For this review, take the finished solid that the model builds, in its own axes (mm). Round coordinates to 2 decimals unless told otherwise and drop trailing zeros. Write each loop counter-clockwise with the first axis right and the second up, starting at its lowest first coordinate (ties: lowest second). Pieces come first, ordered by that corner, then holes. Notation, with made-up numbers: (66.5, 41) - (121.5, 41) arc R28 ccw to (121.5, 60) - close; hole circle Ø3 at (-7, 89). An arc over 180 degrees is marked (long way). One line per item, written item: value. Start each with the question number.
Q1. Add section B-B on z = 3.6. Write out the cut boundary in (x, y).
Q2. Add section C-C on y = 11. Write out the cut boundary in (x, z), and give its area (3 significant figures).
Q3. Add section A-A on x = -15.56. Write out the cut boundary in (y, z), and give its area (3 significant figures).
Q4. Add section D-D on x = -30.56. Write out the cut boundary in (y, z), and give its area (3 significant figures).
Q5. For probe 1 along Y at (x, z) = (32.06, 2.95); probe 2 along X at (y, z) = (6, 2.35); probe 3 along Y at (x, z) = (-30.56, 3.15), list the stretches that pass through material, from the lowest coordinate up.
Q6. Mouldability with a two-part tool opening along Y and no side actions: class faces 1 (the face through (-34.65, 11.99, 2.41)), 2 (the face through (-34.65, -11.99, 2.41)), 3 (the face through (-32.06, 5.15, 2.41)) as +Y half, -Y half, draft (parallel to the pull), parting line (faces both ways), or undercut.
```python
from build123d import *

# Parameters (mm, degrees)
ESQUISSE1_W             = 75
ESQUISSE1_H             = 30
BOSS_EXTRU_1_DEPTH      = 4.7625
CONG_1_R                = 10
ESQUISSE3_R             = 1.5
ENL_V_MAT_EXTRU_3_DEPTH = 10


with BuildPart() as part:
    # Esquisse1 → Boss.-Extru.1 (new body)
    with BuildSketch(Plane.XY):
        Rectangle(ESQUISSE1_W, ESQUISSE1_H)
    extrude(amount=BOSS_EXTRU_1_DEPTH)

    # Congé1
    cong_1_edges = [part.edges().sort_by_distance(p)[0] for p in [
        (-37.5, -15, 2.38125),
        (-37.5, 15, 2.38125),
    ]]
    fillet(cong_1_edges, radius=CONG_1_R)

    # Esquisse3 → Enlèv. mat.-Extru.3 (cut)
    with BuildSketch(Plane.XY.offset(4.7625)):
        with Locations((-15.56, 5.08)):
            Circle(ESQUISSE3_R)
        with Locations((-15.56, -5.08)):
            Circle(ESQUISSE3_R)
        with Locations((32.06, -5.08)):
            Circle(ESQUISSE3_R)
        with Locations((32.06, 5.08)):
            Circle(ESQUISSE3_R)
        with Locations((-30.56, 5.08)):
            Circle(ESQUISSE3_R)
        with Locations((-30.56, -5.08)):
            Circle(ESQUISSE3_R)
    extrude(amount=-ENL_V_MAT_EXTRU_3_DEPTH, mode=Mode.SUBTRACT)


solid = part.part
```
Result set:
1. outline: (-37.5, -5) arc R10 ccw to (-27.5, -15) - (37.5, -15) - (37.5, 15) - (-27.5, 15) arc R10 ccw to (-37.5, 5) - close; hole circle Ø3 at (-30.56, -5.08); hole circle Ø3 at (-30.56, 5.08); hole circle Ø3 at (-15.56, -5.08); hole circle Ø3 at (-15.56, 5.08); hole circle Ø3 at (32.06, -5.08); hole circle Ø3 at (32.06, 5.08)
2. outline: (-35.5, 0) - (37.5, 0) - (37.5, 4.76) - (-35.5, 4.76) - close
2. area: 348 mm^2
3. outline: (-15, 0) - (-6.58, 0) - (-6.58, 4.76) - (-15, 4.76) - close; (-3.58, 0) - (3.58, 0) - (3.58, 4.76) - (-3.58, 4.76) - close; (6.58, 0) - (15, 0) - (15, 4.76) - (6.58, 4.76) - close
3. area: 114 mm^2
4. outline: (-14.52, 0) - (-6.58, 0) - (-6.58, 4.76) - (-14.52, 4.76) - close; (-3.58, 0) - (3.58, 0) - (3.58, 4.76) - (-3.58, 4.76) - close; (6.58, 0) - (14.52, 0) - (14.52, 4.76) - (6.58, 4.76) - close
4. area: 110 mm^2
5. probe 1: y = -15 to -6.58, -3.58 to 3.58, 6.58 to 15
5. probe 2: x = -37.45 to -31.74, -29.38 to -16.74, -14.38 to 30.88, 33.24 to 37.5
5. probe 3: y = -14.52 to -6.58, -3.58 to 3.58, 6.58 to 14.52
6. face 1: +Y half
6. face 2: -Y half
6. face 3: undercut
